```python
from build123d import *

# Parameters (mm, degrees)
LOFT6_OUTLINE_W     = 20
LOFT6_OUTLINE_H     = 19
LOFT6_DEPTH         = 3
LOFT6_DRAFT         = 18.4349488
SKETCH4_W           = 22
SKETCH4_H           = 21
BOSS_EXTRUDE1_DEPTH = 2
SHELL1_T            = -1
SKETCH5_R           = 3.5
SKETCH5_R_2         = 2.5
BOSS_EXTRUDE2_DEPTH = 9.2
SKETCH5_2_R         = 2.5
CUT_EXTRUDE1_DEPTH  = 9.2
SKETCH6_R           = 4
SKETCH6_R_2         = 2.5
CUT_EXTRUDE3_DEPTH  = 0.8


# Read off the part's stored shape, not the designer's step: Loft6
with BuildPart() as part:
    # Loft6 outline → Loft6 (with draft: the straight prism first)
    with BuildSketch(Plane.XY.offset(3)):
        with Locations((0, -4.5)):
            Rectangle(LOFT6_OUTLINE_W, LOFT6_OUTLINE_H)
    extrude(amount=-LOFT6_DEPTH)
    # Loft6: the draft: its side faces are tilted about the plane it starts from
    loft6_sides = [part.faces().sort_by_distance(p)[0] for p in [
        (10, -4.5, 1.5),
        (0, 5, 1.5),
        (-10, -4.5, 1.5),
        (0, -14, 1.5),
    ]]
    draft(loft6_sides, Plane.XY.offset(3), LOFT6_DRAFT)

    # Sketch4 → Boss-Extrude1 (add)
    with BuildSketch(Plane(origin=(0, 0, 0), x_dir=(-1, 0, 0), z_dir=(0, 0, -1))):
        with Locations((0, -4.5)):
            Rectangle(SKETCH4_W, SKETCH4_H)
    extrude(amount=BOSS_EXTRUDE1_DEPTH)

    # Shell1
    shell1_openings = [part.faces().sort_by_distance(p)[0] for p in [
        (0, -4.5, -2),
    ]]
    offset(amount=SHELL1_T, openings=shell1_openings, kind=Kind.INTERSECTION)

    # Sketch5 → Boss-Extrude2 (add)
    # profile 1 of 4: a face of its own
    with BuildSketch(Plane.XY.offset(3)):
        with Locations((-5, 0.666820713)):
            Circle(SKETCH5_R)
        with Locations((-5, 0.666820713)):
            Circle(SKETCH5_R_2, mode=Mode.SUBTRACT)
    # profile 2 of 4: a face of its own
    with BuildSketch(Plane.XY.offset(3)):
        with Locations((5, 0.666820713)):
            Circle(SKETCH5_R)
        with Locations((5, 0.666820713)):
            Circle(SKETCH5_R_2, mode=Mode.SUBTRACT)
    # profile 3 of 4: a face of its own
    with BuildSketch(Plane.XY.offset(3)):
        with Locations((-5, -9.333179287)):
            Circle(SKETCH5_R)
        with Locations((-5, -9.333179287)):
            Circle(SKETCH5_R_2, mode=Mode.SUBTRACT)
    # profile 4 of 4: a face of its own
    with BuildSketch(Plane.XY.offset(3)):
        with Locations((5, -9.333179287)):
            Circle(SKETCH5_R)
        with Locations((5, -9.333179287)):
            Circle(SKETCH5_R_2, mode=Mode.SUBTRACT)
    extrude(amount=-BOSS_EXTRUDE2_DEPTH)

    # Sketch5<2> → Cut-Extrude1 (cut)
    with BuildSketch(Plane.XY.offset(3)):
        with Locations((-5, 0.666820713)):
            Circle(SKETCH5_2_R)
        with Locations((5, 0.666820713)):
            Circle(SKETCH5_2_R)
        with Locations((5, -9.333179287)):
            Circle(SKETCH5_2_R)
        with Locations((-5, -9.333179287)):
            Circle(SKETCH5_2_R)
    extrude(amount=-CUT_EXTRUDE1_DEPTH, mode=Mode.SUBTRACT)

    # Sketch6 → Cut-Extrude3 (cut)
    # profile 1 of 4: a face of its own
    with BuildSketch(Plane.XY.offset(3)):
        with Locations((-5, 0.666820713)):
            Circle(SKETCH6_R)
        with Locations((-5, 0.666820713)):
            Circle(SKETCH6_R_2, mode=Mode.SUBTRACT)
    # profile 2 of 4: a face of its own
    with BuildSketch(Plane.XY.offset(3)):
        with Locations((5, 0.666820713)):
            Circle(SKETCH6_R)
        with Locations((5, 0.666820713)):
            Circle(SKETCH6_R_2, mode=Mode.SUBTRACT)
    # profile 3 of 4: a face of its own
    with BuildSketch(Plane.XY.offset(3)):
        with Locations((5, -9.333179287)):
            Circle(SKETCH6_R)
        with Locations((5, -9.333179287)):
            Circle(SKETCH6_R_2, mode=Mode.SUBTRACT)
    # profile 4 of 4: a face of its own
    with BuildSketch(Plane.XY.offset(3)):
        with Locations((-5, -9.333179287)):
            Circle(SKETCH6_R)
        with Locations((-5, -9.333179287)):
            Circle(SKETCH6_R_2, mode=Mode.SUBTRACT)
    extrude(amount=-CUT_EXTRUDE3_DEPTH, mode=Mode.SUBTRACT)


solid = part.part
```
Geometry: final body of the model. Coordinates: model frame, mm. A direction names the side the tool comes from. Give positions to 0.01 mm unless a question says otherwise; leave off trailing zeros. Loops run counter-clockwise (first coordinate to the right, second up) from the corner with the lowest first, then second, coordinate; pieces in that order, holes last. Notation, with made-up numbers: (46.25, 35.25) -> (57.25, 35.25) arc R10 cw to (57.25, 54.25) -> close; hole circle Ø4 at (-15, 4.25). An arc over 180 degrees is marked (long way). Use one line per item in the form item = value.
Item 1: Section query B-B on y = -4. Output: boundary loops of the cut face in (x, z).
A:
outline = (-11, -2) -> (-10, -2) -> (-10, -0.16) -> (-9.28, 2) -> (9.28, 2) -> (10, -0.16) -> (10, -2) -> (11, -2) -> (11, 0) -> (10, 3) -> (-10, 3) -> (-11, 0) -> close
Item 2: Draft query along Y for faces 1 (the face through (0.9, -14.6, -2)), 2 (the face through (-0.2, -14.5, 1.5)), 3 (the face through (-5.867, -3.238, 2.606)), 4 (the face through (0, 5, -1)). Return one class per face: pulls with the +Y half, pulls with the -Y half, needs draft (parallel to the pull), parting line crosses it, or undercut.
A:
face_1 = needs draft
face_2 = pulls with the -Y half
face_3 = undercut
face_4 = undercut
Item 3: Line query: probe 1 along Y at (x, z) = (5, -4); probe 2 along X at (y, z) = (-3, -1.5); probe 3 along Y at (x, z) = (1.25, -1). Output: solid intervals per line, ascending.
A:
probe_1 = -12.83 to -11.83, -6.83 to -5.83, -2.83 to -1.83, 3.17 to 4.17
probe_2 = -11 to -10, 10 to 11
probe_3 = -15 to -14, 5 to 6
Item 4: Pin query (flat end, axial travel): P1, Ø6.5, axis at x = 5, y = -9.33, coming from the +Z side; P2, Ø4.5, axis at x = 5, y = 0.67, coming from the +Z side. Return the tip coordinate at first contact, or that it passes through.
A:
P1 = 2.2
P2 = through
Item 5: Section query A-A on z = 0.5. Give the number of separate pieces and of enclosed holes in the cut face, and give its area (3 significant figures).
A:
separate_pieces = 5
enclosed_holes = 5
area = 160 mm^2
Item 6: Access query for faces 5 (the face through (-3, 3, 2.2)), 6 (the face through (0, -14, -1)), 7 (the face through (7.3, -0.8, -6.2)). Directions: +Z, -Z, +X, -X, +Y, -Y. A direction counts if a zero-diameter tool reaches every point of the face in a straight line with its end or side. Return the directions, or none.
A:
face_5 = +Z
face_6 = -Z
face_7 = -Z, +X, -X, +Y, -Y
